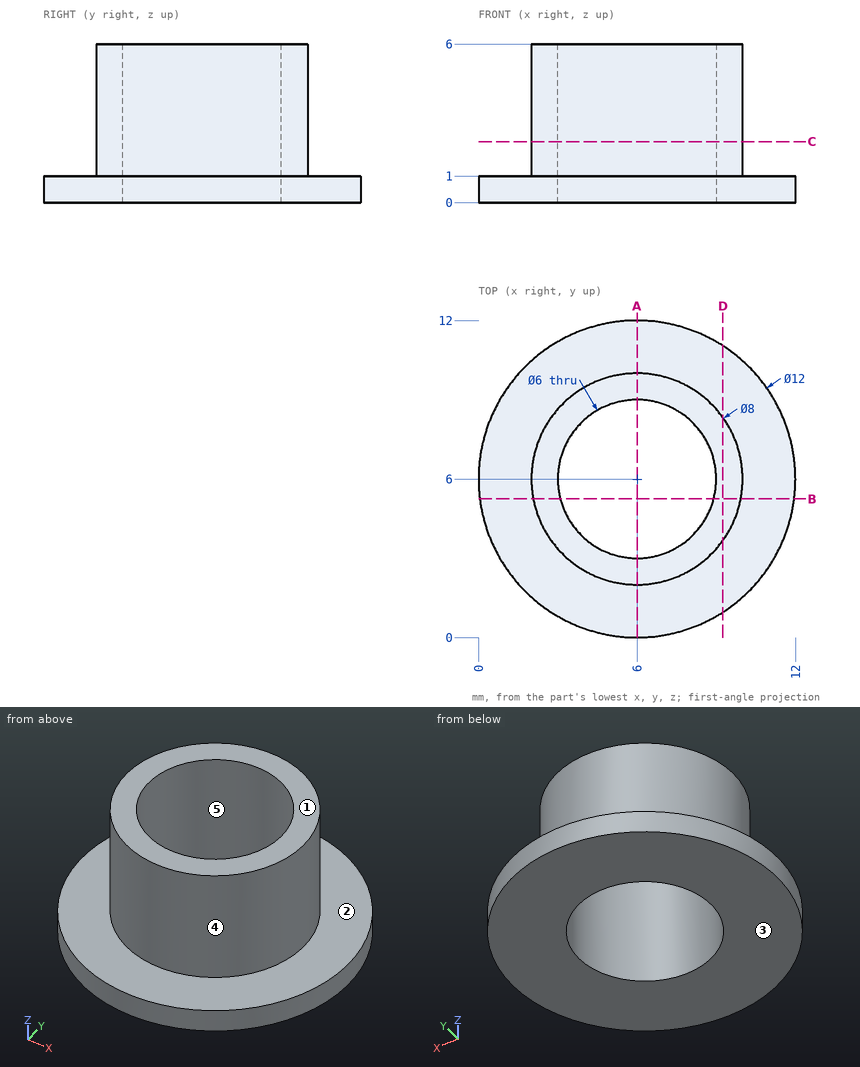
For this review, use the dimensioned drawing (mm, ordinates from the lowest corner) and the shaded views. A direction names the side the tool comes from. Give positions to 0.01 mm unless a question says otherwise; leave off trailing zeros. Loops run counter-clockwise (first coordinate to the right, second up) from the corner with the lowest first, then second, coordinate; pieces in that order, holes last.
Item 1: Take a section at B-B, the plane y = 5.25. State the section outline as (x, z) points.
Item 2: Take a section at D-D, the plane x = 9.25. State the section outline as (y, z) points.
Item 3: Insertion check: pin 1 (2 mm diameter, centred on y = 2, z = 1.5, fed in from -X); pin 2 (3 mm diameter, centred on x = 3.5, z = 2, fed in from -Y). Each pin has a flat end and moves straight along its axis. Give the tip position at first contact, or say it passes through.
Item 4: Take a section at C-C, the plane z = 2.3. State the section outline as (x, y) points.
Item 5: Tool access review of the marked faces 1 and 2: name each direction out of +Z, -Z, +X, -X, +Y, -Y from which nothing blocks a thin tool from reaching the whole face with its end or side.
Item 6: For line 1 along Y through (x, z) = (6, 1.7); line 2 along Y through (x, z) = (6, 0.8); line 3 along Z through (x, y) = (9.75, 2.5), list the stretches that pass through material, from the lowest coordinate up.
Item 7: Draft analysis for pull direction Y (two halves, no side actions). For the marked faces 3, 4 and 5, state which applies: +Y half, -Y half, draft (parallel to the pull), parting line (faces both ways), or undercut.
Item 8: Take a section at A-A, the plane x = 6. State the section outline as (y, z) points.
Calculated:
1. outline: (0.05, 0) - (3.1, 0) - (3.1, 6) - (2.07, 6) - (2.07, 1) - (0.05, 1) - close; (8.9, 0) - (11.95, 0) - (11.95, 1) - (9.93, 1) - (9.93, 6) - (8.9, 6) - close
2. outline: (0.96, 0) - (11.04, 0) - (11.04, 1) - (8.33, 1) - (8.33, 6) - (3.67, 6) - (3.67, 1) - (0.96, 1) - close
3. pin 1: stops at x = 0.88
3. pin 2: stops at y = 0.16
4. outline: circle Ø8 at (6, 6); hole circle Ø6 at (6, 6)
5. face 1: +Z, +X, -X, +Y, -Y
5. face 2: +Z
6. line 1: y = 2 to 3, 9 to 10
6. line 2: y = 0 to 3, 9 to 12
6. line 3: z = 0 to 1
7. face 3: draft
7. face 4: parting line
7. face 5: undercut
8. outline: (0, 0) - (3, 0) - (3, 6) - (2, 6) - (2, 1) - (0, 1) - close; (9, 0) - (12, 0) - (12, 1) - (10, 1) - (10, 6) - (9, 6) - close
